The listing builds one solid part. Answer for the finished solid, in the listing's coordinates (mm). Face numbers are marked on the shaded views. A direction names the side the tool comes from. Give positions to 0.01 mm unless a question says otherwise; leave off trailing zeros. Write each loop counter-clockwise with the first axis right and the second up, starting at its lowest first coordinate (ties: lowest second). Pieces come first, ordered by that corner, then holes. Notation, with made-up numbers: (78.25, -13) - (130.25, -13) arc R22 ccw to (130.25, -7) - close; hole circle Ø3 at (24.25, 1). An arc over 180 degrees is marked (long way). Return JSON: item names as keys, results as strings.
from build123d import *

# Parameters (mm, degrees)
SKETCH005_R     = 11
SKETCH005_R_2   = 6
PAD005_DEPTH    = 1
SKETCH006_R     = 2.5
PAD006_DEPTH    = 14.5
SKETCH001_W     = 41
SKETCH001_H     = 41
PAD001_DEPTH    = 18
CHAMFER_SIZE    = 7.5
FILLET_R        = 2
PAD_DEPTH       = 11
FILLET001_R     = 4
CHAMFER001_SIZE = 1.5
FILLET002_R     = 1
FILLET003_R     = 1
SKETCH002_W     = 41
SKETCH002_H     = 41
PAD002_DEPTH    = 8
FILLET004_R     = 4
SKETCH004_W     = 41
SKETCH004_H     = 41
SKETCH004_R     = 1.3
SKETCH004_R_2   = 6
PAD004_DEPTH    = 1.5
FILLET005_R     = 4
SKETCH003_R     = 16.5
PAD003_DEPTH    = 4


with BuildPart() as pad005:
    # Sketch005 → Pad005 (new body)
    with BuildSketch(Plane.XY.offset(42.5)):
        with Locations((20.5, 20.5)):
            Circle(SKETCH005_R)
        with Locations((20.5, 20.5)):
            Circle(SKETCH005_R_2, mode=Mode.SUBTRACT)
    extrude(amount=PAD005_DEPTH)


with BuildPart() as pad006:
    # Sketch006 → Pad006 (new body)
    with BuildSketch(Plane.XY.offset(41)):
        with Locations((20.5, 20.5)):
            Circle(SKETCH006_R)
    extrude(amount=PAD006_DEPTH)


with BuildPart() as fillet_body:
    # Sketch001 → Pad001 (new body)
    with BuildSketch(Plane.XY.offset(11)):
        with Locations((20.5, 20.5)):
            Rectangle(SKETCH001_W, SKETCH001_H)
    extrude(amount=PAD001_DEPTH)

    # Chamfer
    chamfer_edges = [fillet_body.edges().sort_by_distance(p)[0] for p in [
        (0, 41, 20),
        (41, 41, 20),
        (41, 0, 20),
        (0, 0, 20),
    ]]
    chamfer(chamfer_edges, length=CHAMFER_SIZE)

    # Fillet
    fillet_edges = [fillet_body.edges().sort_by_distance(p)[0] for p in [
        (33.5, 0, 20),
        (41, 7.5, 20),
        (7.5, 0, 20),
        (0, 7.5, 20),
        (0, 33.5, 20),
        (7.5, 41, 20),
        (33.5, 41, 20),
        (41, 33.5, 20),
    ]]
    fillet(fillet_edges, radius=FILLET_R)


with BuildPart() as fillet003:
    # Sketch → Pad (new body)
    with BuildSketch(Plane.XY):
        Polygon((0, 41), (0, 0), (41, 0), (41, 41), (35, 41), (35, 43), (6, 43), (6, 41), align=None)
    extrude(amount=PAD_DEPTH)

    # Fillet001
    fillet001_edges = [fillet003.edges().sort_by_distance(p)[0] for p in [
        (0, 0, 5.5),
        (41, 0, 5.5),
        (0, 41, 5.5),
        (41, 41, 5.5),
    ]]
    fillet(fillet001_edges, radius=FILLET001_R)

    # Chamfer001
    chamfer001_edges = [fillet003.edges().sort_by_distance(p)[0] for p in [
        (6, 43, 5.5),
        (35, 43, 5.5),
    ]]
    chamfer(chamfer001_edges, length=CHAMFER001_SIZE)

    # Fillet002
    fillet002_edges = [fillet003.edges().sort_by_distance(p)[0] for p in [
        (33.5, 43, 5.5),
        (7.5, 43, 5.5),
    ]]
    fillet(fillet002_edges, radius=FILLET002_R)

    # Fillet003
    fillet003_edges = [fillet003.edges().sort_by_distance(p)[0] for p in [
        (35, 41.5, 5.5),
        (6, 41.5, 5.5),
    ]]
    fillet(fillet003_edges, radius=FILLET003_R)


with BuildPart() as fillet004:
    # Sketch002 → Pad002 (new body)
    with BuildSketch(Plane.XY.offset(29)):
        with Locations((20.5, 20.5)):
            Rectangle(SKETCH002_W, SKETCH002_H)
    extrude(amount=PAD002_DEPTH)

    # Fillet004
    fillet004_edges = [fillet004.edges().sort_by_distance(p)[0] for p in [
        (0, 41, 33),
        (41, 41, 33),
        (0, 0, 33),
        (41, 0, 33),
    ]]
    fillet(fillet004_edges, radius=FILLET004_R)


with BuildPart() as fillet005:
    # Sketch004 → Pad004 (new body)
    with BuildSketch(Plane.XY.offset(41)):
        with Locations((20.5, 20.5)):
            Rectangle(SKETCH004_W, SKETCH004_H)
        with Locations((4.5, 35.5)):
            Circle(SKETCH004_R, mode=Mode.SUBTRACT)
        with Locations((35.5, 35.5)):
            Circle(SKETCH004_R, mode=Mode.SUBTRACT)
        with Locations((4.5, 4.5)):
            Circle(SKETCH004_R, mode=Mode.SUBTRACT)
        with Locations((35.5, 4.5)):
            Circle(SKETCH004_R, mode=Mode.SUBTRACT)
        with Locations((20.5, 20.5)):
            Circle(SKETCH004_R_2, mode=Mode.SUBTRACT)
    extrude(amount=PAD004_DEPTH)

    # Fillet005
    fillet005_edges = [fillet005.edges().sort_by_distance(p)[0] for p in [
        (41, 0, 41.75),
        (41, 41, 41.75),
        (0, 0, 41.75),
        (0, 41, 41.75),
    ]]
    fillet(fillet005_edges, radius=FILLET005_R)


with BuildPart() as fusion:
    # Sketch003 → Pad003 (new body)
    with BuildSketch(Plane.XY.offset(37)):
        with Locations((20, 20)):
            Circle(SKETCH003_R)
    extrude(amount=PAD003_DEPTH)

    # Fusion: union Pad005, Pad006, Fillet body, Fillet003, Fillet004, Fillet005
    add(pad005.part)
    add(pad006.part)
    add(fillet_body.part)
    add(fillet003.part)
    add(fillet004.part)
    add(fillet005.part)


solid = fusion.part
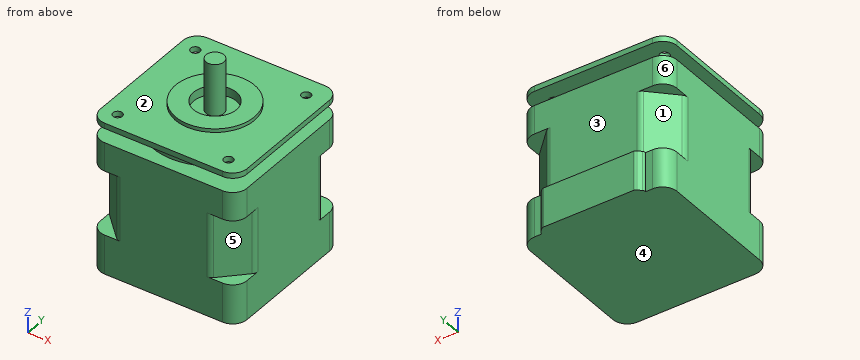
Item 1: Flat-ended cylindrical pins translate along their axes: P1, Ø4, axis at x = 4.5, y = 35.5, coming from the +Z side; P2, Ø3, axis at x = 21.5, z = 31, coming from the +Y side. Find the tip coordinate at first contact, or state that the pin passes through.
Answer below:
{"P1": "stops at z = 42.5", "P2": "stops at y = 41"}
Item 2: The mould has two halves that part along Z. Classify the marked faces 4, 5 and 6: +Z half, -Z half, draft (parallel to the pull), parting line (faces both ways), or undercut.
Answer below:
{"face 4": "-Z half", "face 5": "undercut", "face 6": "draft"}
Item 3: Consider L1, parallel to Y at x = 4.5, z = 42.1; L2, parallel to Z at x = 4, y = 28; L3, parallel to Y at x = 20.5, z = 41.8. Determine where each line is inside the solid, lowest interval first.
Answer below:
{"L1": "y = 0 to 3.2, 5.8 to 34.2, 36.8 to 41", "L2": "z = 0 to 37, 41 to 42.5", "L3": "y = 0 to 14.5, 18 to 23, 26.5 to 41"}
Item 4: A cutting plane is placed at D-D on x = 20.5. Determine the outline of the cut face in (y, z), then the cut area to 3 significant figures.
Answer below:
{"outline": "(0, 0) - (43, 0) - (43, 11) - (41, 11) - (41, 37) - (36.49, 37) - (36.49, 41) - (41, 41) - (41, 42.5) - (31.5, 42.5) - (31.5, 43.5) - (26.5, 43.5) - (26.5, 41) - (23, 41) - (23, 55.5) - (18, 55.5) - (18, 41) - (14.5, 41) - (14.5, 43.5) - (9.5, 43.5) - (9.5, 42.5) - (0, 42.5) - (0, 41) - (3.51, 41) - (3.51, 37) - (0, 37) - close", "area": "1,800 mm²"}
Item 5: A cutting plane is placed at A-A on y = 35.5. Determine the outline of the cut face in (x, z).
Answer below:
{"outline": "(0, 0) - (41, 0) - (41, 11) - (39, 11) - (39, 29) - (41, 29) - (41, 37) - (25.66, 37) - (25.66, 41) - (34.2, 41) - (34.2, 42.5) - (5.8, 42.5) - (5.8, 41) - (14.34, 41) - (14.34, 37) - (0, 37) - (0, 29) - (2, 29) - (2, 11) - (0, 11) - close; (0, 41) - (3.2, 41) - (3.2, 42.5) - (0, 42.5) - close; (36.8, 41) - (41, 41) - (41, 42.5) - (36.8, 42.5) - close"}
Item 6: A cutting plane is placed at B-B on z = 31. Determine the outline of the cut face in (x, y).
Answer below:
{"outline": "(0, 4) arc R4 ccw to (4, 0) - (37, 0) arc R4 ccw to (41, 4) - (41, 37) arc R4 ccw to (37, 41) - (4, 41) arc R4 ccw to (0, 37) - close"}
Item 7: For the marked faces 1, 2 and 3, determine the directions among +Z, -Z, +X, -X, +Y, -Y from which every point of the face is accessible in a straight line to the end or side of a thin tool.
Answer below:
{"face 1": "-X, +Y", "face 2": "+Z", "face 3": "+Z, +X, -X, +Y"}
Item 8: A cutting plane is placed at C-C on y = 30. Determine the outline of the cut face in (x, z).
Answer below:
{"outline": "(0, 0) - (41, 0) - (41, 37) - (33.12, 37) - (33.12, 41) - (41, 41) - (41, 42.5) - (26.05, 42.5) - (26.05, 43.5) - (14.95, 43.5) - (14.95, 42.5) - (0, 42.5) - (0, 41) - (6.88, 41) - (6.88, 37) - (0, 37) - close"}
